Solid Edge part; units mm, degrees
sketch "Sketch1" plane through (0, 0, 0) normal (1, 0, 0) x (0, 1, 0)
  line L0 (0, 0) -> (0, 25.4)
  line L1 (0, 25.4) -> (9.525, 25.4)
  line L2 (9.525, 25.4) -> (9.525, 0)
  line L3 (9.525, 0) -> (0, 0)
  dimension "D1" = 9.525
extrude "ExtrudedProtrusion_1" add sketch "Sketch1" along normal blind 6.35 and the other way blind 168.275
hole "Hole_1" at (-57.15, 0, 12.7) direction (0, 1, 0) diameter 6.35 end through all
hole "Hole1" at (-149.225, 0, 12.7) direction (0, 1, 0) diameter 6.35 end through all
hole "Hole2" at (-57.15, 4.7625, 25.4) direction (0, 0, -1) diameter 3.9675 end up to next
hole "Hole3" at (-149.225, 4.7625, 25.4) direction (0, 0, -1) diameter 3.9675 end up to next
hole "Hole_3" at (-31.75, 4.7625, 25.4) direction (0, 0, -1) diameter 3.9675 end through all
sketch "Sketch2" plane through (0, 12.7, 25.4) normal (0, 0, 1) x (1, 0, 0)
  line L0 (-49.2125, -3.175) -> (-14.2875, -3.175)
  line L1 (-14.2875, -3.175) -> (-14.2875, -12.7)
  line L2 (-14.2875, -12.7) -> (-49.2125, -12.7)
  line L3 (-49.2125, -12.7) -> (-49.2125, -3.175)
  dimension "D1" = 49.2125
extrude "ExtrudedCutout_1" cut sketch "Sketch2" against normal blind 6.35
sketch "Sketch3" plane through (3.0755, 4.7625, 13.1794) normal (0.9659, 0, -0.2588) x (0, 1, 0)
  line L0 (-4.7625, 12.7) -> (-4.7625, -12.7)
  line L1 (-4.7625, -12.7) -> (4.7625, -12.7)
  line L2 (4.7625, -12.7) -> (4.7625, 12.7)
  line L3 (4.7625, 12.7) -> (-4.7625, 12.7)
  dimension "D1" = 4.7625
  dimension "D2" = 4.7625
extrude "ExtrudedProtrusion_2" add sketch "Sketch3" along normal blind 177.8
hole "Hole_4" at (174.8171, 4.7625, -32.8386) direction (-0.9659, 0, 0.2588) diameter 3.9675 depth 25.4
hole "Hole4" at (176.7236, 4.7625, -25.7236) direction (-0.9659, 0, 0.2588) diameter 6.35 depth 25.4
hole "Hole5" at (172.9107, 4.7625, -39.9536) direction (-0.9659, 0, 0.2588) diameter 6.35 depth 25.4
sketch "Sketch4" plane through (4.9146, 0, -9.8296) normal (0, -1, 0) x (1, 0, 0)
  line L0 (1.4479, 35.2763) -> (50.517, 22.1283)
  line L1 (50.517, 22.1283) -> (-23.952, 35.2296)
  line L2 (-23.952, 35.2296) -> (1.4479, 35.2763)
  dimension "D1" = 1.4479
  dimension "D2" = 23.952
extrude "Cutout1" cut sketch "Sketch4" against normal up to next
properties part number "SR-01" material "Aluminum, 1060"
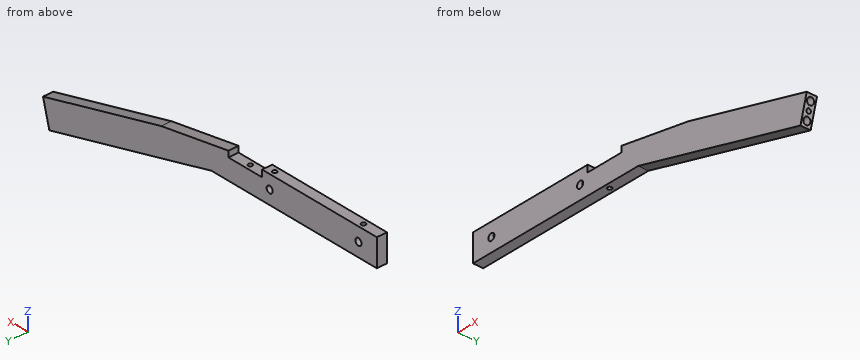
Check sheet for the modelled part. Datum: model origin and axes. Units: mm. Give positions to 0.01 mm unless a question says otherwise; leave off trailing zeros. Write each loop counter-clockwise with the first axis right and the second up, starting at its lowest first coordinate (ties: lowest second). Pieces come first, ordered by that corner, then holes. Notation, with made-up numbers: (62.5, -18.75) -> (96.5, -18.75) arc R23 cw to (96.5, 14.25) -> close; hole circle Ø9 at (-27, -16). An arc over 180 degrees is marked (long way). Write item = value, one per line.
Item 1: Sectioned sample at A-A on x = -22. Record the boundary of the cut face in (y, z) (3 decimals).
Output:
outline = (0, 0) -> (9.525, 0) -> (9.525, 19.05) -> (0, 19.05) -> close
Item 2: Sectioned sample at B-B on x = 82. Record the boundary of the cut face in (y, z) (3 decimals), and give its area (3 significant figures).
Output:
outline = (0, -21.116) -> (9.525, -21.116) -> (9.525, 5.18) -> (0, 5.18) -> close
area = 250 mm^2
Item 3: Gauge pin test, flat ends, axial feed: pin 1 (10 mm diameter, centred on x = -149.225, z = 12.7, fed in from +Y) (3 decimals); pin 2 (3 mm diameter, centred on x = -31.75, y = 4.76, fed in from -Z); pin 3 (4 mm diameter, centred on x = 17, y = 2, fed in from +Z); pin 4 (1 mm diameter, centred on x = 65.5, y = 2.5, fed in from -Z). Record the tip position at first contact, or that the pin passes through.
Output:
pin_1 = 9.525
pin_2 = through
pin_3 = 19.41
pin_4 = -16.83
Item 4: Scan lines: probe 1 along Y at (x, z) = (-57, 18) (3 decimals); probe 2 along Z at (x, y) = (-57.15, 6.5) (3 decimals); probe 3 along Z at (x, y) = (-31.5, 8.5). Record each from-to range of solid material in increasing order. Write a range as from..to.
Output:
probe_1 = 0..2.784, 6.741..9.525
probe_2 = 0..9.525
probe_3 = 0..19.05
